```python
from build123d import *

# Parameters (mm, degrees)
FRONT_SKETCH_R      = 1.905
BOSS_EXTRUDE1_DEPTH = 50.8
CUT_EXTRUDE1_START  = -53.34
CUT_EXTRUDE1_DEPTH  = 48.26
CUT_EXTRUDE2_DEPTH  = 274.638700861
SKETCH3_R           = 3.175
CUT_EXTRUDE3_DEPTH  = 18.03621965
SKETCH4_W           = 50.8
SKETCH4_H           = 19.05
CUT_EXTRUDE4_DEPTH  = 22.86


with BuildPart() as part:
    # front_sketch → Boss-Extrude1 (new body)
    with BuildSketch(Plane(origin=(0, 0, 0), x_dir=(1, 0, 0), z_dir=(0, 1, 0))):
        with BuildLine():
            Line((-94.961375831, 124.478458264), (-121.345326632, 110.234521439))
            ThreePointArc((-121.345326632, 110.234521439), (-122.32001306, 109.300728329), (-122.678671172, 107.99944144))
            Line((-122.678671172, 107.99944144), (-122.678671172, 48.810796684))
            Line((-122.678671172, 48.810796684), (-140.250849959, 48.810796684))
            Line((-140.250849959, 48.810796684), (-140.250849959, -56.645199257))
            Line((-140.250849959, -56.645199257), (-119.167015715, -56.645199257))
            Line((-119.167015715, -56.645199257), (-119.167015715, -126.112255785))
            Line((-119.167015715, -126.112255785), (-95.601645083, -136.460242597))
            Line((-95.601645083, -136.460242597), (-95.601645083, -142.810242597))
            Line((-95.601645083, -142.810242597), (-105.798207048, -142.810242597))
            ThreePointArc((-105.798207048, -142.810242597), (-119.167015715, -139.007347839), (-128.532661201, -128.737404395))
            ThreePointArc((-128.532661201, -128.737404395), (-157.286213724, -5.861503432), (-127.918775374, 116.869125935))
            ThreePointArc((-127.918775374, 116.869125935), (-118.556014486, 127.058910858), (-105.241228699, 130.828458264))
            Line((-105.241228699, 130.828458264), (-94.961375831, 130.828458264))
            Line((-94.961375831, 130.828458264), (-94.961375831, 124.478458264))
        make_face()
        with Locations((-131.296368682, 71.963600743)):
            Circle(FRONT_SKETCH_R, mode=Mode.SUBTRACT)
        with Locations((-131.296368682, -86.786399257)):
            Circle(FRONT_SKETCH_R, mode=Mode.SUBTRACT)
    extrude(amount=BOSS_EXTRUDE1_DEPTH)

    # Sketch1 → Cut-Extrude1 (cut)
    with BuildSketch(Plane(origin=(0, 50.8, 0), x_dir=(1, 0, 0), z_dir=(0, 1, 0)).offset(CUT_EXTRUDE1_START)):
        Polygon((-122.678671172, 48.810796684), (-122.678671172, 107.99944144), (-138.833286115, 78.405119062), (-140.250849959, 48.810796684), align=None)
        Polygon((-119.167015715, -56.645199257), (-140.250849959, -56.645199257), (-139.542068037, -96.192486205), (-119.167015715, -126.112255785), align=None)
    extrude(amount=CUT_EXTRUDE1_DEPTH, mode=Mode.SUBTRACT)

    # Sketch2 → Cut-Extrude2 (cut, through all)
    with BuildSketch(Plane.XY.offset(142.810242597)):
        Polygon((-94.961375831, 0), (-157.287069608, 0), (-157.287069608, 10.05650125), align=None)
    extrude(amount=-CUT_EXTRUDE2_DEPTH, mode=Mode.SUBTRACT)

    # Sketch3 → Cut-Extrude3 (cut, through all)
    with BuildSketch(Plane(origin=(-140.250849959, 0, 0), x_dir=(0, 0, -1), z_dir=(1, 0, 0))):
        with Locations((-17.312177426, 23.984839343)):
            Circle(SKETCH3_R)
        with Locations((11.274067854, 23.984839343)):
            Circle(SKETCH3_R)
    extrude(amount=-CUT_EXTRUDE3_DEPTH, mode=Mode.SUBTRACT)

    # Sketch4 → Cut-Extrude4 (cut)
    with BuildSketch(Plane(origin=(-140.250849959, 0, 0), x_dir=(0, 0, -1), z_dir=(1, 0, 0))):
        with Locations((-3.8461352, 23.892272696)):
            Rectangle(SKETCH4_W, SKETCH4_H)
    extrude(amount=-CUT_EXTRUDE4_DEPTH, mode=Mode.SUBTRACT)


solid = part.part
```
Geometry: final body of the model. Coordinates: model frame, mm. A direction names the side the tool comes from. Coordinates: 2 decimals unless noted, no trailing zeros. Order: outer loops, then holes, each group sorted by start corner. A loop starts at its lowest first (then second) coordinate and runs counter-clockwise, first axis right, second up.
Item 1: Draft query along Z for faces 1 (the face through (-95.602, 25, 140)), 2 (the face through (-122.679, 48, -79)), 3 (the face through (-157.285, 37.848, 7.644)). Return one class per face: released by +Z, released by -Z, zero draft, split by the parting line, or undercut.
Answer:
face 1: zero draft
face 2: undercut
face 3: split by the parting line
Item 2: Contact query for flat-ended pins moving along their axis: P1, Ø2.5, axis at y = 47.5, z = -76, coming from the +X side; P2, Ø1, axis at y = 31, z = 2, coming from the -X side; P3, Ø1.5, axis at x = -125.5, y = 48.5, coming from the -Z side; P4, Ø1.5, axis at x = -128.5, y = 49.5, coming from the +Z side. Output: stop coordinate, or through.
Answer:
P1: stops at x = -122.68
P2: passes through
P3: stops at z = -121.69
P4: stops at z = 130.19
Item 3: Section query A-A (y = 25.5). Output: boundary loops of the cut face in (x, z).
Answer:
outline: (-156.35, 29.25) - (-140.25, 29.25) - (-140.25, 56.65) - (-139.54, 96.19) - (-119.17, 126.11) - (-95.6, 136.46) - (-95.6, 142.81) - (-105.8, 142.81) arc R25.4 ccw to (-128.53, 128.74) arc R274 ccw to start; (-155.84, -21.55) arc R274 ccw to (-127.92, -116.87) arc R25.4 ccw to (-105.24, -130.83) - (-94.96, -130.83) - (-94.96, -124.48) - (-121.35, -110.23) arc R2.54 cw to (-122.68, -108) - (-138.83, -78.41) - (-140.25, -48.81) - (-140.25, -21.55) - close
Item 4: Section query B-B (x = -102). Output: boundary loops of the cut face in (y, z), then the cut area to 3 significant figures.
Answer:
outline: (1.14, -130.83) - (50.8, -130.83) - (50.8, -120.68) - (1.14, -120.68) - close; (1.14, 133.65) - (50.8, 133.65) - (50.8, 142.81) - (1.14, 142.81) - close
area: 959 mm2
Item 5: Section query D-D (y = 41). Output: boundary loops of the cut face in (x, z).
Answer:
outline: (-140.25, -48.81) - (-140.25, 56.65) - (-139.54, 96.19) - (-119.17, 126.11) - (-95.6, 136.46) - (-95.6, 142.81) - (-105.8, 142.81) arc R25.4 ccw to (-128.53, 128.74) arc R274 ccw to (-127.92, -116.87) arc R25.4 ccw to (-105.24, -130.83) - (-94.96, -130.83) - (-94.96, -124.48) - (-121.35, -110.23) arc R2.54 cw to (-122.68, -108) - (-138.83, -78.41) - close
Item 6: Access query for faces 4 (the face through (-129.5, 24.52, 110.94)), 5 (the face through (-148, 24, -21.554)), 6 (the face through (-107.969, 25.044, -117.456)). Directions: +Z, -Z, +X, -X, +Y, -Y. A direction counts if a zero-diameter tool reaches every point of the face in a straight line with its end or side. Return the directions, or none.
Answer:
face 4: +X, -Y
face 5: +X, -X
face 6: +X, +Y, -Y
Item 7: Material intervals for line 1 along X through (y, z) = (22, -22); line 2 along Z through (x, y) = (-121.5, 22.5); line 3 along Y through (x, z) = (-120, 93), sorted ascending.
Answer:
line 1: x = -155.8 to -140.25
line 2: z = -124.94 to -110.14, 122.69 to 137.38
line 3: y = 45.72 to 50.8
Item 8: Section query C-C (z = 0.5). Output: boundary loops of the cut face in (x, y), then the cut area to 3 significant figures.
Answer:
outline: (-157.22, 10.05) - (-140.25, 7.31) - (-140.25, 14.37) - (-157.22, 14.37) - close; (-157.22, 33.42) - (-140.25, 33.42) - (-140.25, 50.8) - (-157.22, 50.8) - close
area: 392 mm2
